```python
from build123d import *

# Parameters (mm, degrees)
SKETCH1_R                  = 107.5
SKETCH1_R_2                = 94
BOSS_EXTRUDE1_DEPTH        = 10
F_10_0_10_DIAMETER_HOLE1_D = 10
F_6_0_6_DIAMETER_HOLE1_D   = 6
M4_TAPPED_HOLE2_D          = 3.3
SKETCH15_R                 = 45
CUT_EXTRUDE1_DEPTH         = 4
SKETCH16_R                 = 15
CUT_EXTRUDE2_DEPTH         = 2


with BuildPart() as part:
    # Sketch1 → Boss-Extrude1 (new body)
    with BuildSketch(Plane.XY):
        Circle(SKETCH1_R)
        Circle(SKETCH1_R_2, mode=Mode.SUBTRACT)
        Circle(SKETCH1_R_2)
    extrude(amount=BOSS_EXTRUDE1_DEPTH)

    # Ø10.0 (10) Diameter Hole1 (through all)
    with Locations(Plane.XY.offset(10)):
        with Locations((-30.310889132, 17.5), (-30.310889132, -17.5), (0, -35), (30.310889132, -17.5), (30.310889132, 17.5), (0, 35)):
            Hole(F_10_0_10_DIAMETER_HOLE1_D / 2)

    # Ø6.0 (6) Diameter Hole1 (through all)
    with Locations(Plane.XY.offset(10)):
        with Locations((-87.468565782, -50.5), (-94.018248613, -36.899443461), (-98.46771913, -22.47461433), (-100.717583515, -7.547739452), (-100.717583515, 7.547739452), (-98.46771913, 22.47461433), (-94.018248613, 36.899443461), (-87.468565782, 50.5), (0, 101), (15.053268884, 99.871913449), (29.770272616, 96.512853384), (43.822257651, 90.997855658), (56.895325864, 83.450116206), (68.697446515, 74.038239055), (78.964979729, 62.972469988), (87.468565782, 50.5), (87.468565782, -50.5), (78.964979729, -62.972469988), (68.697446515, -74.038239055), (56.895325864, -83.450116206), (43.822257651, -90.997855658), (29.770272616, -96.512853384), (15.053268884, -99.871913449), (0, -101)):
            Hole(F_6_0_6_DIAMETER_HOLE1_D / 2)

    # M4 Tapped Hole2 (through all)
    with Locations(Plane.XY.offset(10)):
        with Locations((-58.820508076, 61.880108514), (-24.179491924, 81.880108514), (-12.179491924, 61.095498823), (-46.820508076, 41.095498823), (12.5, 21.650635095), (-25, 0), (12.5, -21.650635095), (59, 20), (83, 20), (59, -20), (83, -20), (-12.179491924, -61.095498823), (-46.820508076, -41.095498823), (-58.820508076, -61.880108514), (-24.179491924, -81.880108514), (-8, 0), (0, 8), (8, 0), (0, -8)):
            Hole(M4_TAPPED_HOLE2_D / 2)

    # Sketch15 → Cut-Extrude1 (cut)
    with BuildSketch(Plane(origin=(0, 0, 0), x_dir=(-1, 0, 0), z_dir=(0, 0, -1))):
        Circle(SKETCH15_R)
    extrude(amount=-CUT_EXTRUDE1_DEPTH, mode=Mode.SUBTRACT)

    # Sketch16 → Cut-Extrude2 (cut)
    with BuildSketch(Plane(origin=(0, 0, 4), x_dir=(-1, 0, 0), z_dir=(0, 0, -1))):
        Circle(SKETCH16_R)
    extrude(amount=-CUT_EXTRUDE2_DEPTH, mode=Mode.SUBTRACT)


solid = part.part
```
CAD build for the part. Positions are in the model's coordinates, mm. A direction names the side the tool comes from. Give positions to 0.01 mm unless a question says otherwise; leave off trailing zeros. Write each question's results on one line, items separated by ' | '.
1. Which spindle directions (+Z, -Z, +X, -X, +Y, -Y) get a long thin tool onto all of the face, cutting with end or side? Do faces 3 (the cylindrical face through (81.176, 65, 4.93)), 4 (the flat face through (0, 0, 6)). Say none if no direction does.
Geometry check:
face 3: +Z, -Z | face 4: -Z
2. Drop flat-ended pins along their axis: P1, Ø13, axis at x = -30.31, y = 17.5, coming from the -Z side; P2, Ø3.5, axis at x = 87.47, y = -50.5, coming from the -Z side; P3, Ø4.5, axis at x = 8, y = 0, coming from the -Z side; P4, Ø5, axis at y = -60.5, z = 1.5, coming from the -X side. Give the stop position or say it passes through.
Geometry check:
P1: z = 4 | P2: through | P3: z = 6 | P4: x = -90.51
3. Cut at A-A, the plane z = 8. Give the number of separate pieces and of enclosed holes in the cut face, then the cut area to 3 significant figures.
Geometry check:
separate pieces: 1 | enclosed holes: 49 | area: 35,000 mm²
4. Two-plate mould, pull along X, no slides. Class faces 1 (the flat face through (-2, 2, 10)), 2 (the cylindrical face through (-85.26, 52.53, 4.93)): pulls with the +X half, pulls with the -X half, needs draft (parallel to the pull), parting line crosses it, or undercut.
Geometry check:
face 1: needs draft | face 2: undercut
5. Wall check: probe 1 along Y at (x, z) = (-96.5, 6.75); probe 2 along X at (y, z) = (-51.5, 2); probe 3 along X at (y, z) = (49, 5.75). Give the ranges that are in metal, low to high. Write a range as [from, to].
Geometry check:
probe 1: [-47.37, -38.58], [-35.21, -24.74], [-20.21, 20.21], [24.74, 35.21], [38.58, 47.37] | probe 2: [-94.36, -90.3], [-84.64, 84.64], [90.3, 94.36] | probe 3: [-95.68, -90.07], [-84.87, 84.87], [90.07, 95.68]
